Geometry check sheet. Reference: the model listing, model coordinates, mm. A direction names the side the tool comes from. Give positions to 0.01 mm unless a question says otherwise; leave off trailing zeros. Order: outer loops, then holes, each group sorted by start corner. A loop starts at its lowest first (then second) coordinate and runs counter-clockwise, first axis right, second up. Notation, with made-up numbers: (87.25, -20) - (111.25, -20) arc R22 cw to (111.25, -14) - close; hole circle Ø7 at (86.25, 13.25). An arc over 180 degrees is marked (long way). Put each result on its own line as item: value. Start each with the question number.
```python
from build123d import *

# Parameters (mm, degrees)
SKETCH1_W           = 444.5
SKETCH1_H           = 508
BOSS_EXTRUDE1_DEPTH = 6.35
SKETCH2_W           = 88.9
SKETCH2_H           = 60.452
CUT_EXTRUDE1_DEPTH  = 230.886
SKETCH3_R           = 2.667
CUT_EXTRUDE2_DEPTH  = 230.886


with BuildPart() as part:
    # Sketch1 → Boss-Extrude1 (new, symmetric)
    with BuildSketch(Plane(origin=(0, 0, 0), x_dir=(1, 0, 0), z_dir=(0, 1, 0))):
        Rectangle(SKETCH1_W, SKETCH1_H)
    extrude(amount=BOSS_EXTRUDE1_DEPTH, both=True)

    # Sketch2 → Cut-Extrude1 (cut)
    with BuildSketch(Plane(origin=(0, 6.35, 0), x_dir=(1, 0, 0), z_dir=(0, 1, 0))):
        with Locations((-177.8, 223.774)):
            Rectangle(SKETCH2_W, SKETCH2_H)
    cut_extrude1 = extrude(amount=-CUT_EXTRUDE1_DEPTH, mode=Mode.SUBTRACT)

    # Mirror1: Cut-Extrude1 across plane
    add(cut_extrude1.mirror(Plane.XY), mode=Mode.SUBTRACT)

    # Sketch3 → Cut-Extrude2 (cut)
    with BuildSketch(Plane(origin=(0, 6.35, 0), x_dir=(1, 0, 0), z_dir=(0, 1, 0))):
        with Locations(Location((199.898, -241.3, 0), (0, 0, 270))):
            Circle(SKETCH3_R)
        with Locations(Location((199.898, 241.3, 0), (0, 0, 270))):
            Circle(SKETCH3_R)
    extrude(amount=-CUT_EXTRUDE2_DEPTH, mode=Mode.SUBTRACT)


solid = part.part
```
Item 1: Gauge pin test, flat ends, axial feed: pin 1 Ø4 at (x, y) = (-183.5, -1.5) entering from -Z; pin 2 Ø6.5 at (x, y) = (-184, -3) entering from +Z. Record the tip position at first contact, or that the pin passes through.
Item 2: Thickness scan on line 1 along X through (y, z) = (-1.75, 241.3) (3 decimals); line 2 along Z through (x, y) = (198, 4.75); line 3 along X through (y, z) = (0.25, -197). Record the ranges inside material, lowest first.
Item 3: Set-up check for faces 1 (the face through (42, 0, -254)), 2 (the face through (-133.35, 0, 223)), 3 (the face through (-178, 0, -193.548)): record each of +Z, -Z, +X, -X, +Y, -Y from which the full face is reachable in a straight line by a thin tool's end or side.
Item 4: Cross-section at B-B (x = -180). Enter the section's corners in (y, z).
Item 5: Cross-section at A-A (y = -3.5). Enter the section's corners in (x, z), and give its area (3 significant figures).
Recorded:
1. pin 1: stops at z = -193.55
1. pin 2: stops at z = 193.55
2. line 1: x = -133.35 to 197.231, 202.565 to 222.25
2. line 2: z = -254 to -243.17, -239.43 to 239.43, 243.17 to 254
2. line 3: x = -133.35 to 222.25
3. face 1: -Z, +X, -X, +Y, -Y
3. face 2: +Z, -X, +Y, -Y
3. face 3: -Z, -X, +Y, -Y
4. outline: (-6.35, -193.55) - (6.35, -193.55) - (6.35, 193.55) - (-6.35, 193.55) - close
5. outline: (-222.25, -193.55) - (-133.35, -193.55) - (-133.35, -254) - (222.25, -254) - (222.25, 254) - (-133.35, 254) - (-133.35, 193.55) - (-222.25, 193.55) - close; hole circle Ø5.33 at (199.9, -241.3); hole circle Ø5.33 at (199.9, 241.3)
5. area: 215,000 mm^2
